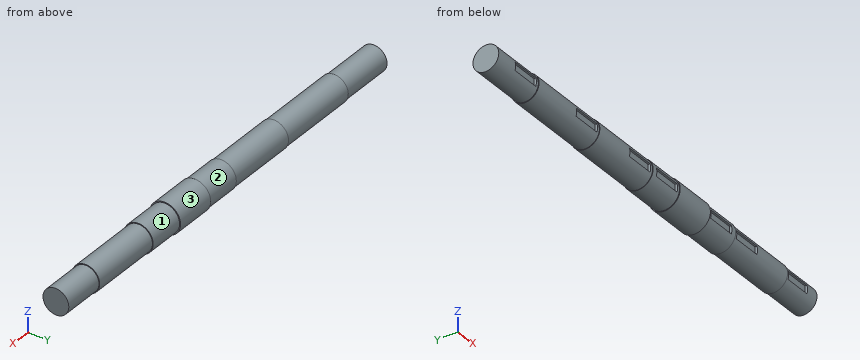
Solid Edge part; units mm, degrees
sketch "Sketch1" plane through (0, 0, 0) normal (0, -1, 0) x (1, 0, 0)
  line L0 (1469.4867, 25) -> (1469.4867, 0)
  line L1 (1469.4867, 0) -> (649.4867, 0)
  line L2 (649.4867, 0) -> (649.4867, 25)
  line L3 (649.4867, 25) -> (729.4867, 25)
  line L4 (729.4867, 25) -> (729.4867, 26.5)
  line L5 (729.4867, 26.5) -> (889.4867, 26.5)
  line L6 (889.4867, 26.5) -> (889.4867, 27.5)
  line L7 (889.4867, 27.5) -> (1029.4867, 27.5)
  line L8 (1029.4867, 27.5) -> (1029.4867, 28.5)
  line L9 (1029.4867, 28.5) -> (1099.4867, 28.5)
  line L10 (1099.4867, 28.5) -> (1099.4867, 30)
  line L11 (1099.4867, 30) -> (1179.4867, 30)
  line L12 (1179.4867, 30) -> (1179.4867, 28)
  line L13 (1179.4867, 28) -> (1249.4867, 28)
  line L14 (1249.4867, 28) -> (1249.4867, 26.5)
  line L15 (1249.4867, 26.5) -> (1389.4867, 26.5)
  line L16 (1389.4867, 26.5) -> (1389.4867, 25)
  line L17 (1389.4867, 25) -> (1469.4867, 25)
revolve "RevolvedProtrusion1" add sketch "Sketch1" angle 360 about axis through (0, 0, 0) along (1, 0, 0)
sketch "Sketch2" plane through (689.4867, -25, 0) normal (0, -1, 0) x (-1, 0, 0)
  line L0 (20, -8) -> (-35, -8)
  line L1 (-35, -8) -> (-35, 0)
  line L2 (-35, 0) -> (-35, 8)
  line L3 (-35, 8) -> (20, 8)
  line L4 (20, 8) -> (20, -8)
extrude "Cutout1" cut sketch "Sketch2" against normal blind 5
sketch "Sketch3" plane through (809.4867, -26.5, 0) normal (0, -1, 0) x (-1, 0, 0)
  line L0 (-75, 0) -> (-75, 8)
  line L1 (-75, 8) -> (-20, 8)
  line L2 (-20, 8) -> (-20, -8)
  line L3 (-20, -8) -> (-75, -8)
  line L4 (-75, -8) -> (-75, 0)
  dimension "D1" = 75
extrude "Cutout2" cut sketch "Sketch3" against normal blind 5
sketch "Sketch4" plane through (959.4867, -27.5, 0) normal (0, -1, 0) x (-1, 0, 0)
  line L0 (-65, 0) -> (-65, 8)
  line L1 (-65, 8) -> (-10, 8)
  line L2 (-10, 8) -> (-10, -8)
  line L3 (-10, -8) -> (-65, -8)
  line L4 (-65, -8) -> (-65, 0)
  dimension "D1" = 65
  dimension "D2" = 10
extrude "Keyway_Thickness" cut sketch "Sketch4" against normal blind 5
sketch "Sketch5" plane through (1064.4867, -28.5, 0) normal (0, -1, 0) x (-1, 0, 0)
  line L0 (-30, 0) -> (-30, 8)
  line L1 (-30, 8) -> (25, 8)
  line L2 (25, 8) -> (25, -8)
  line L3 (25, -8) -> (-30, -8)
  line L4 (-30, -8) -> (-30, 0)
  dimension "D1" = 30
  dimension "D2" = 25
extrude "Cutout3" cut sketch "Sketch5" against normal blind 5
sketch "Sketch6" plane through (1214.4867, -28, 0) normal (0, -1, 0) x (-1, 0, 0)
  line L0 (-25, 0) -> (-25, 8)
  line L1 (-25, 8) -> (30, 8)
  line L2 (30, 8) -> (30, -8)
  line L3 (30, -8) -> (-25, -8)
  line L4 (-25, -8) -> (-25, 0)
  dimension "D1" = 30
  dimension "D2" = 25
extrude "Cutout4" cut sketch "Sketch6" against normal blind 5
sketch "Sketch7" plane through (1319.4867, -26.5, 0) normal (0, -1, 0) x (-1, 0, 0)
  line L0 (65, 0) -> (65, 8)
  line L1 (65, 8) -> (10, 8)
  line L2 (10, 8) -> (10, -8)
  line L3 (10, -8) -> (65, -8)
  line L4 (65, -8) -> (65, 0)
  dimension "D1" = 65
  dimension "D2" = 10
extrude "Cutout5" cut sketch "Sketch7" against normal blind 5
sketch "Sketch8" plane through (1429.4867, -25, 0) normal (0, -1, 0) x (-1, 0, 0)
  line L0 (35, 0) -> (35, 8)
  line L1 (35, 8) -> (-20, 8)
  line L2 (-20, 8) -> (-20, -8)
  line L3 (-20, -8) -> (35, -8)
  line L4 (35, -8) -> (35, 0)
  dimension "D1" = 35
  dimension "D2" = 20
extrude "Cutout6" cut sketch "Sketch8" against normal blind 5
sketch "Sketch9" plane through (1469.4867, 0, 0) normal (1, 0, 0) x (0, 1, 0)
  circle A0 centre (0, 0) radius 25
extrude "Protrusion1" add sketch "Sketch9" against normal blind 25
sketch "Sketch10" plane through (649.4867, 0, 0) normal (-1, 0, 0) x (0, -1, 0)
  circle A0 centre (0, 0) radius 25
extrude "Extruded_for_Bearing_A" add sketch "Sketch10" along normal blind 25
Source: CAD feature listing. Evaluate the final solid. Frame: model axes, mm. Face numbers are marked on the shaded views. A direction names the side the tool comes from. Give positions to 0.01 mm unless a question says otherwise; leave off trailing zeros. Write each loop counter-clockwise with the first axis right and the second up, starting at its lowest first coordinate (ties: lowest second). Pieces come first, ordered by that corner, then holes. Notation, with made-up numbers: M 43,33.25 L 101,33.25 A7 cw 101,37.25 Z; hole C -12,-29.75 d5. An arc over 180 degrees is marked long. Answer as a JSON object with one key per item and string values.
Q1. Ray query, line 1 along X through (y, z) = (-22, -19.5); line 2 along Z through (x, y) = (1054, 1); line 3 along X through (y, z) = (18.5, -18.5). Return the intervals inside material, ascending.
Geometry check:
{"line 1": "x = 1099.49 to 1179.49", "line 2": "z = -28.48 to 28.48", "line 3": "x = 729.49 to 1389.49"}
Q2. Access query for the marked faces 1, 2 and 3. Directions: +Z, -Z, +X, -X, +Y, -Y. A direction counts if a zero-diameter tool reaches every point of the face in a straight line with its end or side. Return the directions, or none.
Geometry check:
{"face 1": "+X", "face 2": "-X", "face 3": "+X, -X"}
Q3. Cut plane C-C, the plane x = 793. Return the cut outline in (y, z).
Geometry check:
{"outline": "C 0,0 d53"}
Q4. Contact query for flat-ended pins moving along their axis: P1, Ø1.9, axis at x = 999, y = -23.5, coming from the -Z side; P2, Ø3, axis at x = 1274, y = 16.5, coming from the +Z side; P3, Ø1.8, axis at x = 1418.5, y = -22, coming from the +Z side; P4, Ø6, axis at y = -18.5, z = 17, coming from the -X side. Output: stop coordinate, or through.
Geometry check:
{"P1": "stops at z = -15.74", "P2": "stops at z = 21.85", "P3": "stops at z = 13.41", "P4": "stops at x = 624.49"}
Q5. Cut plane B-B, the plane x = 913.5. Return the cut outline in (y, z), then the cut area to 3 significant figures.
Geometry check:
{"outline": "C 0,0 d55", "area": "2,380 mm^2"}
